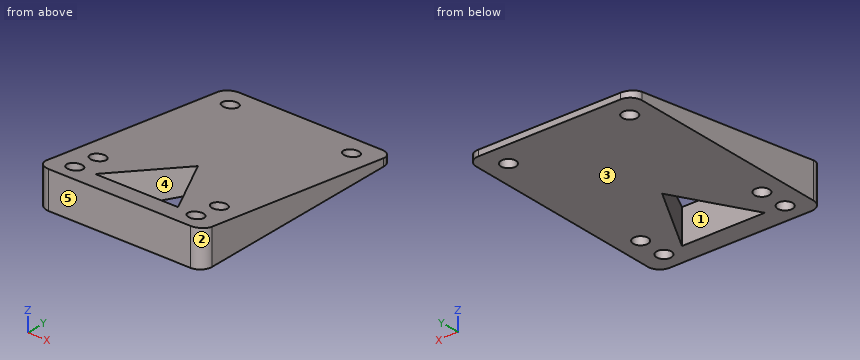
```python
from build123d import *

# Parameters (mm, degrees)
F0_R          = 2.5
F1_DEPTH      = 20
F3_DEPTH      = 25
F5_DEPTH      = 33.15069
F5_DEPTH_BACK = 22.85131


with BuildPart() as f1:
    # F0 (on Top) → F1 (new body)
    with BuildSketch(Plane.XY):
        with BuildLine():
            Line((29.14969, 36.637019), (-18.85031, 36.637019))
            ThreePointArc((-18.85031, 36.637019), (-21.678737, 35.465446), (-22.85031, 32.637019))
            Line((-22.85031, 32.637019), (-22.85031, -37.362981))
            ThreePointArc((-22.85031, -37.362981), (-21.678737, -40.191408), (-18.85031, -41.362981))
            Line((-18.85031, -41.362981), (29.14969, -41.362981))
            ThreePointArc((29.14969, -41.362981), (31.978117, -40.191408), (33.14969, -37.362981))
            Line((33.14969, -37.362981), (33.14969, 32.637019))
            ThreePointArc((33.14969, 32.637019), (31.978117, 35.465446), (29.14969, 36.637019))
        make_face()
        with Locations((-15.35031, -34.862981)):
            Circle(F0_R, mode=Mode.SUBTRACT)
        with Locations((-15.35031, -25.337981)):
            Circle(F0_R, mode=Mode.SUBTRACT)
        with Locations((25.64969, -34.862981)):
            Circle(F0_R, mode=Mode.SUBTRACT)
        with Locations((25.64969, -25.337981)):
            Circle(F0_R, mode=Mode.SUBTRACT)
        with Locations((-15.35031, 28.637019)):
            Circle(F0_R, mode=Mode.SUBTRACT)
        with Locations((25.64969, 28.637019)):
            Circle(F0_R, mode=Mode.SUBTRACT)
    extrude(amount=F1_DEPTH)

    # F2 (on face) → F3 (cut)
    with BuildSketch(Plane.XY.offset(20)):
        Polygon((5.14969, -9.362981), (-8.85031, -34.362981), (19.14969, -34.362981), align=None)
    extrude(amount=-F3_DEPTH, mode=Mode.SUBTRACT)

    # F4 (on Right) → F5 (cut, two sides)
    with BuildSketch(Plane.YZ) as f5_sk:
        Polygon((36.637019, 2), (36.637019, 20), (-41.362981, 20), (-41.362981, 12.5), align=None)
    extrude(amount=F5_DEPTH, mode=Mode.SUBTRACT)
    extrude(f5_sk.sketch, amount=-F5_DEPTH_BACK, mode=Mode.SUBTRACT)


solid = f1.part
```
The model under review builds one solid part; all positions refer to its coordinate system, in mm. Face numbers are marked on the shaded views. A direction names the side the tool comes from. Round coordinates to 2 decimals unless told otherwise and drop trailing zeros. Write each loop counter-clockwise with the first axis right and the second up, starting at its lowest first coordinate (ties: lowest second). Pieces come first, ordered by that corner, then holes.
(1) Mouldability with a two-part tool opening along Y and no side actions: class the marked faces 1, 2 and 3 as +Y half, -Y half, draft (parallel to the pull), parting line (faces both ways), or undercut.
(2) We need section A-A on x = 26.5. Give the boundary of the cut face in (y, z), and give its area (3 significant figures).
(3) We need section C-C on x = 3. Give the boundary of the cut face in (y, z).
(4) Insertion check: pin 1 (8 mm diameter, centred on x = -10.5, y = -28, fed in from +Z); pin 2 (4 mm diameter, centred on x = -15.35, y = 28.64, fed in from -Z); pin 3 (6 mm diameter, centred on x = -15.35, y = -25.34, fed in from +Z). Each pin has a flat end and moves straight along its axis. Give the tip position at first contact, or say it passes through.
(5) We need section D-D on x = -14. Give the boundary of the cut face in (y, z).
(6) Machinability: for the marked faces 4 and 5, which of the approach directions +Z, -Z, +X, -X, +Y, -Y give a long, thin tool a straight path to every point of the face, cutting with its end or side? Answer none if there is none.
(7) We need section B-B on z = 4.75. Give the boundary of the cut face in (x, y).
(8) Wall thickness on L1, parallel to X at y = 29.5, z = 2; L2, parallel to Y at x = -14, z = 3.25; L3, parallel to X at y = -25.5, z = 5.75: over which ranges is each line inside the solid? List them lowest first.
Findings below:
1. face 1: undercut
1. face 2: -Y half
1. face 3: draft
2. outline: (-41.36, 0) - (-37.21, 0) - (-37.21, 11.94) - (-41.36, 12.5) - close; (-32.51, 0) - (-27.69, 0) - (-27.69, 10.66) - (-32.51, 11.31) - close; (-22.99, 0) - (26.29, 0) - (26.29, 3.39) - (-22.99, 10.03) - close; (30.99, 0) - (36.64, 0) - (36.64, 2) - (30.99, 2.76) - close
2. area: 448 mm2
3. outline: (-41.36, 0) - (-34.36, 0) - (-34.36, 11.56) - (-41.36, 12.5) - close; (-13.2, 0) - (36.64, 0) - (36.64, 2) - (-13.2, 8.71) - close
4. pin 1: stops at z = 11.24
4. pin 2: passes through
4. pin 3: stops at z = 10.75
5. outline: (-41.36, 0) - (-36.97, 0) - (-36.97, 11.91) - (-41.36, 12.5) - close; (-32.76, 0) - (-27.44, 0) - (-27.44, 10.63) - (-32.76, 11.34) - close; (-23.23, 0) - (26.53, 0) - (26.53, 3.36) - (-23.23, 10.06) - close; (30.74, 0) - (36.64, 0) - (36.64, 2) - (30.74, 2.79) - close
6. face 4: +Z, -Z
6. face 5: +Z, -Z, +X, -X, -Y
7. outline: (-22.85, -37.36) arc R4 ccw to (-18.85, -41.36) - (29.15, -41.36) arc R4 ccw to (33.15, -37.36) - (33.15, 16.21) - (-22.85, 16.21) - close; hole circle Ø5 at (-15.35, -34.86); hole circle Ø5 at (-15.35, -25.34); hole (-8.85, -34.36) - (19.15, -34.36) - (5.15, -9.36) - close; hole circle Ø5 at (25.65, -34.86); hole circle Ø5 at (25.65, -25.34)
8. L1: x = -22.85 to -17.7, -13 to 23.3, 28 to 33.15
8. L2: y = -41.36 to -36.97, -32.76 to -27.44, -23.23 to 26.53
8. L3: x = -22.85 to -17.85, -12.86 to -3.89, 14.19 to 23.15, 28.14 to 33.15
